```python
from build123d import *

# Parameters (mm, degrees)
SKETCH1_W           = 170.18
SKETCH1_H           = 170.18
SKETCH1_R           = 1.9750024
SKETCH1_R_2         = 1.974999987
BOSS_EXTRUDE1_DEPTH = 15.875
CUT_EXTRUDE1_DEPTH  = 14.300000102
SKETCH4_W           = 86.99999999
SKETCH4_H           = 50.000000076
BOSS_EXTRUDE2_DEPTH = 21.048998796
SKETCH5_R           = 2.325000049
BOSS_EXTRUDE3_DEPTH = 6.99999997


with BuildPart() as part:
    # Sketch1 → Boss-Extrude1 (new body)
    with BuildSketch(Plane(origin=(0, 0, 0), x_dir=(1, 0, 0), z_dir=(0, 1, 0))):
        Rectangle(SKETCH1_W, SKETCH1_H)
        with Locations(Location((-80.01, 78.74, 0), (0, 0, 270))):
            Circle(SKETCH1_R, mode=Mode.SUBTRACT)
        with Locations(Location((74.91000004, 78.74, 0), (0, 0, 270))):
            Circle(SKETCH1_R, mode=Mode.SUBTRACT)
        with Locations(Location((-80.01, -78.74, 0), (0, 0, 270))):
            Circle(SKETCH1_R, mode=Mode.SUBTRACT)
        with Locations(Location((52.07, -78.74, 0), (0, 0, 270))):
            Circle(SKETCH1_R_2, mode=Mode.SUBTRACT)
    extrude(amount=BOSS_EXTRUDE1_DEPTH)

    # Sketch3 → Cut-Extrude1 (cut)
    with BuildSketch(Plane(origin=(0, 15.875, 0), x_dir=(1, 0, 0), z_dir=(0, 1, 0))):
        with BuildLine():
            Line((-76.7588, 78.74), (-76.7588, 85.09))
            Line((-76.7588, 85.09), (-85.09, 85.09))
            Line((-85.09, 85.09), (-85.09, 75.4888))
            Line((-85.09, 75.4888), (-80.01, 75.4888))
            ThreePointArc((-80.01, 75.4888), (-77.711054433, 76.441054433), (-76.7588, 78.74))
        make_face()
        with BuildLine():
            Line((71.65880004, 78.74), (71.65880004, 85.09))
            Line((71.65880004, 85.09), (85.09, 85.09))
            Line((85.09, 85.09), (85.09, 75.4888))
            Line((85.09, 75.4888), (74.91000004, 75.4888))
            ThreePointArc((74.91000004, 75.4888), (72.611054473, 76.441054433), (71.65880004, 78.74))
        make_face()
        with BuildLine():
            Line((48.8188, -78.74), (48.8188, -85.09))
            Line((48.8188, -85.09), (55.3212, -85.09))
            Line((55.3212, -85.09), (55.3212, -78.74))
            ThreePointArc((55.3212, -78.74), (52.07, -75.4888), (48.8188, -78.74))
        make_face()
        with BuildLine():
            Line((-80.01, -75.4888), (-85.09, -75.4888))
            Line((-85.09, -75.4888), (-85.09, -85.09))
            Line((-85.09, -85.09), (-76.7588, -85.09))
            Line((-76.7588, -85.09), (-76.7588, -78.74))
            ThreePointArc((-76.7588, -78.74), (-77.711054433, -76.441054433), (-80.01, -75.4888))
        make_face()
    extrude(amount=-CUT_EXTRUDE1_DEPTH, mode=Mode.SUBTRACT)

    # Sketch4 → Boss-Extrude2 (add)
    with BuildSketch(Plane(origin=(0, 15.875, 0), x_dir=(1, 0, 0), z_dir=(0, 1, 0))):
        with Locations((7.169000013, 28.739999924)):
            Rectangle(SKETCH4_W, SKETCH4_H)
    extrude(amount=BOSS_EXTRUDE2_DEPTH)

    # Sketch5 → Boss-Extrude3 (add)
    with BuildSketch(Plane(origin=(85.09, 0, 0), x_dir=(0, 0, -1), z_dir=(1, 0, 0))):
        with Locations(Location((-64.510000012, 11.574999964, 0), (0, 0, 180))):
            Circle(SKETCH5_R)
        with Locations(Location((-48.009999992, 11.574999964, 0), (0, 0, 180))):
            Circle(SKETCH5_R)
    extrude(amount=BOSS_EXTRUDE3_DEPTH)


solid = part.part
```
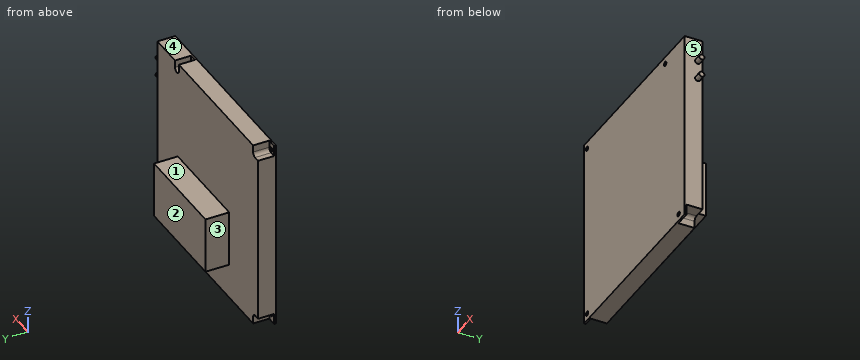
The listing builds one solid part. Answer for the finished solid, in the listing's coordinates (mm). Face numbers are marked on the shaded views. A direction names the side the tool comes from. Round coordinates to 2 decimals unless told otherwise and drop trailing zeros. Write each loop counter-clockwise with the first axis right and the second up, starting at its lowest first coordinate (ties: lowest second). Pieces come first, ordered by that corner, then holes. Notation, with made-up numbers: (80.5, 51.25) -> (87.5, 51.25) arc R16 cw to (87.5, 82.25) -> close; hole circle Ø8 at (16.25, 1.5). An arc over 180 degrees is marked (long way). Write item = value, one per line.
1) Section C-C on x = -33 is taken. Write down the section's boundary in (y, z) (3 decimals), plus the area to 3 significant figures.
Check values:
outline = (0, -85.09) -> (15.875, -85.09) -> (15.875, -53.74) -> (36.924, -53.74) -> (36.924, -3.74) -> (15.875, -3.74) -> (15.875, 85.09) -> (0, 85.09) -> close
area = 3,750 mm²
2) Section B-B on z = -41.5 is taken. Write down the section's boundary in (x, y) (3 decimals), plus the area to 3 significant figures.
Check values:
outline = (-85.09, 0) -> (85.09, 0) -> (85.09, 15.875) -> (50.669, 15.875) -> (50.669, 36.924) -> (-36.331, 36.924) -> (-36.331, 15.875) -> (-85.09, 15.875) -> close
area = 4,530 mm²
3) Straight lines are drawn through the part: line 1 along Z through (x, y) = (-80.01, 1.2) (3 decimals); line 2 along X through (y, z) = (1, 78); line 3 along X through (y, z) = (8.5, 60.5). For each, find the intervals that lie inside material, in ascending order. Write a range as [from, to].
Check values:
line_1 = [-85.09, -80.715], [-76.765, 76.765], [80.715, 85.09]
line_2 = [-85.09, -81.84], [-78.18, 50.24], [53.9, 85.09]
line_3 = [-85.09, 85.09]
4) Given pin 1 (5 mm diameter, centred on y = 12.5, z = -81.5, fed in from -X); pin 2 (3 mm diameter, centred on y = 7.5, z = -82.5, fed in from +X); pin 3 (2.5 mm diameter, centred on x = -82.5, z = 79.5, fed in from +Y) (3 decimals); pin 4 (2.5 mm diameter, centred on x = -80.01, z = 78.74, fed in from -Y), each flat-ended and moving along its own axis, determine where each tip first touches the part or whether it passes through.
Check values:
pin_1 = -76.76
pin_2 = 71.66
pin_3 = 1.575
pin_4 = through
5) Section D-D on z = -64 is taken. Write down the section's boundary in (x, y) (3 decimals), plus the area to 3 significant figures.
Check values:
outline = (-85.09, 0) -> (85.09, 0) -> (85.09, 15.875) -> (-85.09, 15.875) -> close
area = 2,700 mm²
6) Section A-A on y = 5 is taken. Write down the section's boundary in (x, z), plus the area to 3 significant figures.
Check values:
outline = (-85.09, -75.49) -> (-80.01, -75.49) arc R3.25 cw to (-76.76, -78.74) -> (-76.76, -85.09) -> (71.66, -85.09) -> (71.66, -78.74) arc R3.25 cw to (74.91, -75.49) -> (85.09, -75.49) -> (85.09, 85.09) -> (55.32, 85.09) -> (55.32, 78.74) arc R3.25 cw to (48.82, 78.74) -> (48.82, 85.09) -> (-76.76, 85.09) -> (-76.76, 78.74) arc R3.25 cw to (-80.01, 75.49) -> (-85.09, 75.49) -> close
area = 28,600 mm²
7) For a pull along X with two mould halves and no side action, classify the marked faces 3, 4 and 5 as released by +X, released by -X, zero draft, split by the parting line, or undercut.
Check values:
face_3 = released by -X
face_4 = zero draft
face_5 = released by +X
8) Which of the six approach directions +Z, -Z, +X, -X, +Y, -Y give full straight-line access (tool end or side, diameter ignored) to the marked faces 1 and 2?
Check values:
face_1 = +Z, +X, -X, +Y
face_2 = +Z, -Z, +X, -X, +Y
